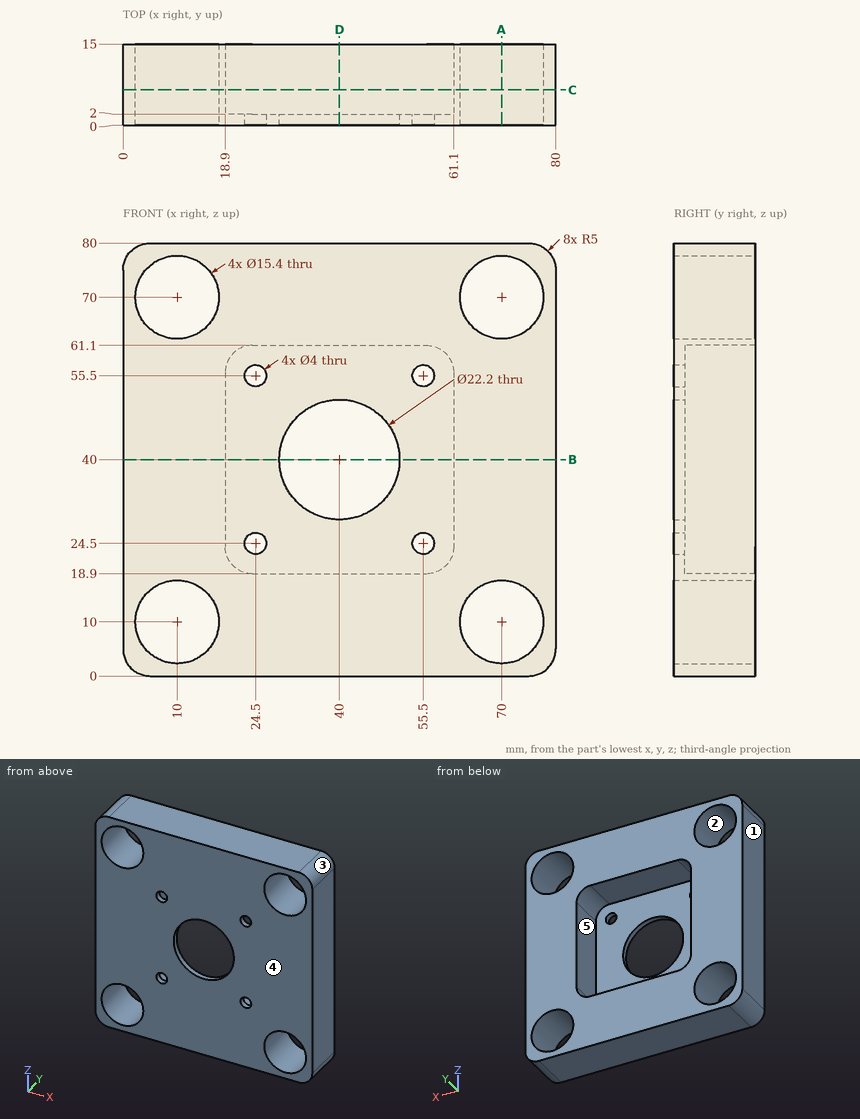
Geometry: see drawing. Coordinates: mm, zero at the bounding-box minimum. A direction names the side the tool comes from. Coordinates: 2 decimals unless noted, no trailing zeros. Order: outer loops, then holes, each group sorted by start corner. A loop starts at its lowest first (then second) coordinate and runs counter-clockwise, first axis right, second up. Notation, with made-up numbers: M 16,67 L 47,67 A7 ccw 47,72 Z; hole C 61,6 d8. An arc over 180 degrees is marked long. Write item = value, one per line. Start each with the question number.
(1) Section C-C on y = 6.5. Output: boundary loops of the cut face in (x, z), and give its area (3 significant figures).
(2) Section A-A on x = 70. Output: boundary loops of the cut face in (y, z).
(3) First-contact query: P1, Ø21, axis at x = 38.5, z = 37.5, coming from the +Y side. Flat tip, straight axial feed; report the tip coordinate or a pass-through.
(4) Pull-direction query (Z, two-part tool) for the marked faces 1, 2 and 3; classes: released by +Z, released by -Z, zero draft, split by the parting line, or undercut.
(5) Section D-D on x = 40. Output: boundary loops of the cut face in (y, z).
(6) Reachability of the marked faces 4 and 5 from +Z, -Z, +X, -X, +Y, -Y: full face, straight path, thin tool, end or side. Return the list, or none.
(7) Section B-B on z = 40. Output: boundary loops of the cut face in (x, y).
(8) Line query: line 1 along Z through (x, y) = (69.5, 5); line 2 along Z through (x, y) = (55.5, 1.45). Output: solid intervals per line, ascending. Write a range as [from, to].
Result set:
q1.outline = M 0,5 A5 ccw 5,0 L 75,0 A5 ccw 80,5 L 80,75 A5 ccw 75,80 L 5,80 A5 ccw 0,75 Z; hole C 10,10 d15.4; hole C 10,70 d15.4; hole M 18.9,23.9 A5 ccw 23.9,18.9 L 56.1,18.9 A5 ccw 61.1,23.9 L 61.1,56.1 A5 ccw 56.1,61.1 L 23.9,61.1 A5 ccw 18.9,56.1 Z; hole C 70,10 d15.4; hole C 70,70 d15.4
q1.area = 3,870 mm²
q2.outline = M 0,0 L 15,0 L 15,2.3 L 0,2.3 Z; M 0,17.7 L 15,17.7 L 15,62.3 L 0,62.3 Z; M 0,77.7 L 15,77.7 L 15,80 L 0,80 Z
q3.P1 = 2
q4.face_1 = zero draft
q4.face_2 = undercut
q4.face_3 = released by +Z
q5.outline = M 0,0 L 15,0 L 15,18.9 L 2,18.9 L 2,28.9 L 0,28.9 Z; M 0,51.1 L 2,51.1 L 2,61.1 L 15,61.1 L 15,80 L 0,80 Z
q6.face_4 = +Z, -Z, +X, -X, -Y
q6.face_5 = +Y
q7.outline = M 0,0 L 28.9,0 L 28.9,2 L 18.9,2 L 18.9,15 L 0,15 Z; M 51.1,0 L 80,0 L 80,15 L 61.1,15 L 61.1,2 L 51.1,2 Z
q8.line_1 = [0, 2.32], [17.68, 62.32], [77.68, 80]
q8.line_2 = [0, 22.5], [26.5, 53.5], [57.5, 80]
